```python
from build123d import *

# Parameters (mm, degrees)
BASE_FLANGE1_OUTLINE_W = 160
BASE_FLANGE1_OUTLINE_H = 10
BASE_FLANGE1_DEPTH     = 280
CUT_EXTRUDE2_DEPTH     = 15
SKETCH16_R             = 8
CUT_EXTRUDE4_DEPTH     = 15


# Read off the part's stored shape, not the designer's step: Base-Flange1
with BuildPart() as part:
    # Base-Flange1 outline → Base-Flange1 (new body)
    with BuildSketch(Plane(origin=(0, 0, 0), x_dir=(1, 0, 0), z_dir=(0, 1, 0))):
        with Locations((80, -5)):
            Rectangle(BASE_FLANGE1_OUTLINE_W, BASE_FLANGE1_OUTLINE_H)
    extrude(amount=BASE_FLANGE1_DEPTH)

    # Sketch12 → Cut-Extrude2 (cut)
    with BuildSketch(Plane.XY.offset(10)):
        Polygon((160, 280), (120, 280), (160, 140), align=None)
        Polygon((0, 280), (40, 280), (0, 140), align=None)
    extrude(amount=-CUT_EXTRUDE2_DEPTH, mode=Mode.SUBTRACT)

    # Sketch16 → Cut-Extrude4 (cut)
    with BuildSketch(Plane.XY.offset(10)):
        with Locations((80, 240)):
            Circle(SKETCH16_R)
        with Locations((80, 160)):
            Circle(SKETCH16_R)
        with Locations((40, 40)):
            Circle(SKETCH16_R)
        with Locations((120, 40)):
            Circle(SKETCH16_R)
    extrude(amount=-CUT_EXTRUDE4_DEPTH, mode=Mode.SUBTRACT)


solid = part.part
```
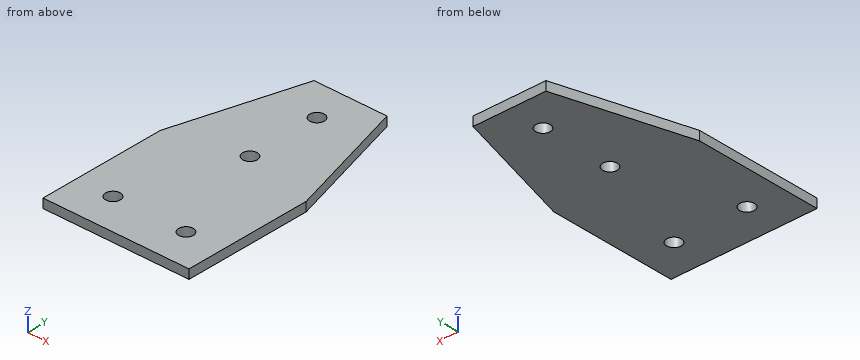
The model under review builds one solid part; all positions refer to its coordinate system, in mm. Coordinates: 2 decimals unless noted, no trailing zeros. Write each loop counter-clockwise with the first axis right and the second up, starting at its lowest first coordinate (ties: lowest second). Pieces come first, ordered by that corner, then holes.
1) To check wall thickness, follow probe 1 along Y at (x, z) = (80, 6); probe 2 along X at (y, z) = (41, 9.75); probe 3 along X at (y, z) = (233.5, 0.5). State the ranges of each line that lie inside material, in increasing order.
2) We need section B-B on z = 6. State the section outline as (x, y) points.
3) We need section A-A on x = 80. State the section outline as (y, z) points.
4) Clearance check with flat-ended pins moving along their axes: pin 1 Ø9.5 at (x, y) = (40, 40) entering from -Z; pin 2 Ø5 at (y, z) = (214.5, 7) entering from +X. State where each tip first meets the part, or that it passes through.
5) We need section D-D on x = 23. State the section outline as (y, z) points.
6) We need section C-C on y = 240. State the section outline as (x, z) points, then the cut area to 3 significant figures.
Answer list:
1. probe 1: y = 0 to 152, 168 to 232, 248 to 280
1. probe 2: x = 0 to 32.06, 47.94 to 112.06, 127.94 to 160
1. probe 3: x = 26.71 to 75.34, 84.66 to 133.29
2. outline: (0, 0) - (160, 0) - (160, 140) - (120, 280) - (40, 280) - (0, 140) - close; hole circle Ø16 at (40, 40); hole circle Ø16 at (80, 160); hole circle Ø16 at (80, 240); hole circle Ø16 at (120, 40)
3. outline: (0, 0) - (152, 0) - (152, 10) - (0, 10) - close; (168, 0) - (232, 0) - (232, 10) - (168, 10) - close; (248, 0) - (280, 0) - (280, 10) - (248, 10) - close
4. pin 1: passes through
4. pin 2: stops at x = 139.43
5. outline: (0, 0) - (220.5, 0) - (220.5, 10) - (0, 10) - close
6. outline: (28.57, 0) - (72, 0) - (72, 10) - (28.57, 10) - close; (88, 0) - (131.43, 0) - (131.43, 10) - (88, 10) - close
6. area: 869 mm2
